from build123d import *

# Parameters (mm, degrees)
EXTRUDE_1_DEPTH     = 5
SKETCH_1_12_R       = 1.5
CUT_EXTRUDE_1_DEPTH = 109.226902848
CUT_EXTRUDE_START   = 5
SKETCH_1_13_R       = 2.25
CUT_EXTRUDE_3_DEPTH = 3
SKETCH_2_R          = 0.75
CUT_EXTRUDE_4_DEPTH = 2
SKETCH_3_R          = 0.75
CUT_EXTRUDE_5_DEPTH = 2
SKETCH_4_R          = 0.75
CUT_EXTRUDE_6_DEPTH = 109.226902848
SKETCH_5_R          = 0.75
CUT_EXTRUDE_7_DEPTH = 2


with BuildPart() as part:
    # 草图1 → 凸台-拉伸1 (new body)
    with BuildSketch(Plane(origin=(0, 0, 0), x_dir=(1, 0, 0), z_dir=(0, 1, 0))):
        Polygon((-25.75, 0), (0, 0), (0, 91.231745931), (-12.313708499, 91.231745931), (-12.313708499, 98.231745931), (0, 98.231745931), (0, 105), (-25.75, 105), align=None)
    extrude(amount=EXTRUDE_1_DEPTH)

    # 草图1<12> → 切除-拉伸1 (cut, through all)
    with BuildSketch(Plane(origin=(0, 0, 0), x_dir=(1, 0, 0), z_dir=(0, 1, 0))):
        with Locations(Location((-20.313708499, 83.231745931, 0), (0, 0, 270))):
            Circle(SKETCH_1_12_R)
        with Locations(Location((-20.313708499, 16.763708499, 0), (0, 0, 270))):
            Circle(SKETCH_1_12_R)
        with Locations(Location((-9, 5.45, 0), (0, 0, 270))):
            Circle(SKETCH_1_12_R)
    extrude(amount=CUT_EXTRUDE_1_DEPTH, mode=Mode.SUBTRACT)

    # 草图1<13> → 切除-拉伸3 (cut)
    with BuildSketch(Plane(origin=(0, 0, 0), x_dir=(1, 0, 0), z_dir=(0, 1, 0)).offset(CUT_EXTRUDE_START)):
        with Locations(Location((-20.313708499, 83.231745931, 0), (0, 0, 270))):
            Circle(SKETCH_1_13_R)
        with Locations(Location((-9, 5.45, 0), (0, 0, 270))):
            Circle(SKETCH_1_13_R)
        with Locations(Location((-20.313708499, 16.763708499, 0), (0, 0, 270))):
            Circle(SKETCH_1_13_R)
    extrude(amount=-CUT_EXTRUDE_3_DEPTH, mode=Mode.SUBTRACT)

    # 草图2 → 切除-拉伸4 (cut)
    with BuildSketch(Plane.XY):
        with Locations((-20.75, 2.5)):
            Circle(SKETCH_2_R)
        with Locations((-5, 2.5)):
            Circle(SKETCH_2_R)
    extrude(amount=-CUT_EXTRUDE_4_DEPTH, mode=Mode.SUBTRACT)

    # 草图3 → 切除-拉伸5 (cut)
    with BuildSketch(Plane(origin=(0, 0, 0), x_dir=(0, 0, -1), z_dir=(1, 0, 0))):
        with Locations((22.5, 2.5)):
            Circle(SKETCH_3_R)
    extrude(amount=-CUT_EXTRUDE_5_DEPTH, mode=Mode.SUBTRACT)

    # 草图4 → 切除-拉伸6 (cut, through all)
    with BuildSketch(Plane(origin=(0, 5, 0), x_dir=(1, 0, 0), z_dir=(0, 1, 0))):
        with Locations(Location((-6, 16, 0), (0, 0, 270))):
            Circle(SKETCH_4_R)
        with Locations(Location((-19.75, 6, 0), (0, 0, 270))):
            Circle(SKETCH_4_R)
    extrude(amount=-CUT_EXTRUDE_6_DEPTH, mode=Mode.SUBTRACT)

    # 草图5 → 切除-拉伸7 (cut)
    with BuildSketch(Plane.ZY.offset(25.75)):
        with Locations((-10, 2.5)):
            Circle(SKETCH_5_R)
        with Locations((-50, 2.5)):
            Circle(SKETCH_5_R)
        with Locations((-70, 2.5)):
            Circle(SKETCH_5_R)
        with Locations((-90, 2.5)):
            Circle(SKETCH_5_R)
        with Locations((-30, 2.5)):
            Circle(SKETCH_5_R)
    extrude(amount=-CUT_EXTRUDE_7_DEPTH, mode=Mode.SUBTRACT)


solid = part.part
The listing builds one solid part. Answer for the finished solid, in the listing's coordinates (mm). A direction names the side the tool comes from. Round coordinates to 2 decimals unless told otherwise and drop trailing zeros. Write each loop counter-clockwise with the first axis right and the second up, starting at its lowest first coordinate (ties: lowest second). Pieces come first, ordered by that corner, then holes. Notation, with made-up numbers: (23.5, -18) - (35.5, -18) arc R17 cw to (35.5, -5) - close; hole circle Ø11 at (-15, -19.75). An arc over 180 degrees is marked (long way). Use one line per item in the form item = value. Start each with the question number.
Item 1: Determine the mould class of faces 1 (the cylindrical face through (-18.42, 3.52, -15.55)), 2 (the flat face through (-13, 5, -53)), 3 (the cylindrical face through (-7.48, 3.52, -7.11)), 4 (the flat face through (0, 2, -45)) for opening direction X: +X half, -X half, draft (parallel to the pull), parting line (faces both ways), or undercut.
Item 2: Find the intervals of material crossed by line 1 (Z direction, x = -24.5, y = 2.4); line 2 (Z direction, x = -5.5, y = 3); line 3 (Z direction, x = -7.5, y = 4.8), in increasing order. Write a range as [from, to].
Item 3: A cutting plane is placed at A-A (x = -9). Write down the section's boundary in (y, z).
Item 4: A cutting plane is placed at B-B (z = -83.5). Write down the section's boundary in (x, y), plus the area to 3 significant figures.
Item 5: A cutting plane is placed at C-C (y = 4.05). Write down the section's boundary in (x, z).
Item 6: A tool of negligible diameter and unlimited length cuts with its end or side. For faces 5 (the flat face through (-12.314, 2, -95)), 6 (the flat face through (-22, 2, -83)), 7 (the cylindrical face through (-9.91, 0.99, -6.64)), from which of +Z, -Z, +X, -X, +Y, -Y can it reach the whole face along a straight path? Write none if from no direction.
Item 7: Flat-ended cylindrical pins translate along their axes: pin 1 Ø4 at (x, z) = (-9, -5.45) entering from +Y; pin 2 Ø5 at (x, z) = (-9, -5.45) entering from +Y; pin 3 Ø1.3 at (x, z) = (-9, -5.5) entering from +Y; pin 4 Ø1.2 at (y, z) = (2.5, -70) entering from -X. Find the tip coordinate at first contact, or state that the pin passes through.
The answers:
q1.face_1 = undercut
q1.face_2 = draft
q1.face_3 = undercut
q1.face_4 = +X half
q2.line_1 = [-105, -90.74], [-89.26, -70.74], [-69.26, -50.74], [-49.26, -30.74], [-29.26, -10.74], [-9.26, 0]
q2.line_2 = [-105, -98.23], [-91.23, -16.56], [-15.44, -2]
q2.line_3 = [-105, -98.23], [-91.23, -7.13], [-3.77, 0]
q3.outline = (0, -105) - (5, -105) - (5, -98.23) - (0, -98.23) - close; (0, -91.23) - (5, -91.23) - (5, -7.7) - (2, -7.7) - (2, -6.95) - (0, -6.95) - close; (0, -3.95) - (2, -3.95) - (2, -3.2) - (5, -3.2) - (5, 0) - (0, 0) - close
q4.outline = (-25.75, 0) - (-21.79, 0) - (-21.79, 2) - (-22.55, 2) - (-22.55, 5) - (-25.75, 5) - close; (-18.84, 0) - (0, 0) - (0, 5) - (-18.08, 5) - (-18.08, 2) - (-18.84, 2) - close
q4.area = 109 mm^2
q5.outline = (-25.75, -105) - (0, -105) - (0, -98.23) - (-12.31, -98.23) - (-12.31, -91.23) - (0, -91.23) - (0, 0) - (-25.75, 0) - close; hole circle Ø4.5 at (-20.31, -83.23); hole circle Ø4.5 at (-20.31, -16.76); hole circle Ø1.5 at (-19.75, -6); hole circle Ø4.5 at (-9, -5.45); hole circle Ø1.5 at (-6, -16)
q6.face_5 = +X, +Y, -Y
q6.face_6 = +Y
q6.face_7 = +Y, -Y
q7.pin_1 = 2
q7.pin_2 = 5
q7.pin_3 = through
q7.pin_4 = -23.75
